Geometry: final body of the model. Coordinates: model frame, mm. Face numbers are marked on the shaded views. Give positions to 0.01 mm unless a question says otherwise; leave off trailing zeros. Write each loop counter-clockwise with the first axis right and the second up, starting at its lowest first coordinate (ties: lowest second). Pieces come first, ordered by that corner, then holes.
from build123d import *

# Parameters (mm, degrees)
F0_W     = 25.9
F0_H     = 9.85
F0_W_2   = 4.5
F0_H_2   = 4.5
F1_DEPTH = 5
F2_DEPTH = 4.08
F2_TAPER = 0.5
F3_W     = 3.15
F3_H     = 9.85
F4_DEPTH = 1
F5_R     = 2


with BuildPart() as f1:
    # F0 (on Front) → F1 (new body)
    with BuildSketch(Plane.XZ):
        with Locations((-28.4469606161, 4.925)):
            Rectangle(F0_W, F0_H)
        with Locations((-32.7639606161, 4.925)):
            Rectangle(F0_W_2, F0_H_2, mode=Mode.SUBTRACT)
        with Locations((-24.1299606161, 4.925)):
            Rectangle(F0_W_2, F0_H_2, mode=Mode.SUBTRACT)
        with Locations((-24.1299606161, 4.925)):
            Rectangle(F0_W_2, F0_H_2)
        with Locations((-32.7639606161, 4.925)):
            Rectangle(F0_W_2, F0_H_2)
    extrude(amount=F1_DEPTH)


with BuildPart() as f1b:
    # F0 (on Front) → F1, piece 2 (new body)
    with BuildSketch(Plane.XZ):
        with Locations((0.6030393839, 4.925)):
            Rectangle(F0_W, F0_H)
        with Locations((-3.7139606161, 4.925)):
            Rectangle(F0_W_2, F0_H_2, mode=Mode.SUBTRACT)
        with Locations((4.9200393839, 4.925)):
            Rectangle(F0_W_2, F0_H_2, mode=Mode.SUBTRACT)
        with Locations((4.9200393839, 4.925)):
            Rectangle(F0_W_2, F0_H_2)
        with Locations((-3.7139606161, 4.925)):
            Rectangle(F0_W_2, F0_H_2)
    extrude(amount=F1_DEPTH)


with BuildPart() as f2_tool:
    # F0 (on Front) → F2 (new body)
    with BuildSketch(Plane.XZ):
        with Locations((4.9200393839, 4.925)):
            Rectangle(F0_W_2, F0_H_2)
        with Locations((-3.7139606161, 4.925)):
            Rectangle(F0_W_2, F0_H_2)
        with Locations((-24.1299606161, 4.925)):
            Rectangle(F0_W_2, F0_H_2)
        with Locations((-32.7639606161, 4.925)):
            Rectangle(F0_W_2, F0_H_2)
    extrude(amount=F2_DEPTH, taper=F2_TAPER)


with BuildPart() as f1_1:
    add(f1.part)

    # F2: cut by f2_tool
    add(f2_tool.part, mode=Mode.SUBTRACT)



with BuildPart() as f1b_1:
    add(f1b.part)

    # F2: cut by f2_tool
    add(f2_tool.part, mode=Mode.SUBTRACT)


with BuildPart() as f1_2:
    add(f1_1.part)

    add(f1b_1.part)  # F4 merges F1b
    # F3 (on face) → F4 (join)
    with BuildSketch(Plane.XZ.offset(5)):
        with Locations((-13.9219606161, 4.925)):
            Rectangle(F3_W, F3_H)
    extrude(amount=-F4_DEPTH)

    # F5
    f5_edges = [f1_2.edges().sort_by_distance(p)[0] for p in [
        (-12.346961, 0, 4.925),
        (-15.496961, 0, 4.925),
        (13.553039, 0, 4.925),
        (-41.396961, 0, 4.925),
    ]]
    fillet(f5_edges, radius=F5_R)


solid = f1_2.part
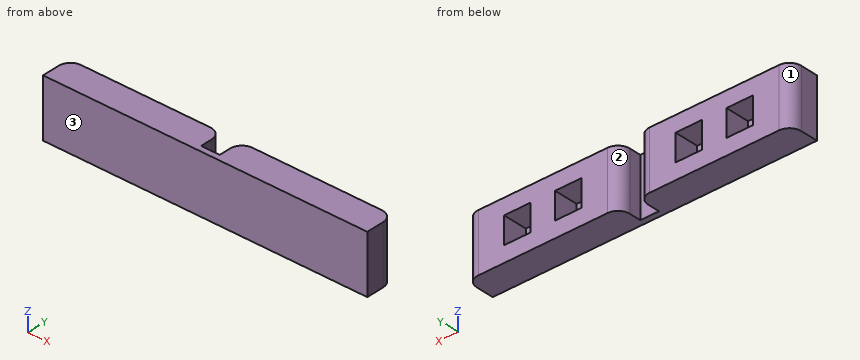
Q1. Pull-direction query (X, two-part tool) for the marked faces 1, 2 and 3; classes: released by +X, released by -X, zero draft, split by the parting line, or undercut.
Filled sheet:
face 1: released by -X
face 2: undercut
face 3: zero draft
Q2. Section C-C on x = -16.5. Output: boundary loops of the cut face in (y, z), plus the area to 3 significant figures.
Filled sheet:
outline: (-5, 0) - (-0.27, 0) - (-0.27, 9.85) - (-5, 9.85) - close
area: 46.6 mm2
Q3. Section A-A on z = 8. Output: boundary loops of the cut face in (x, y), plus the area to 3 significant figures.
Filled sheet:
outline: (-41.4, -5) - (13.55, -5) - (13.55, -2) arc R2 ccw to (11.55, 0) - (-10.35, 0) arc R2 ccw to (-12.35, -2) - (-12.35, -4) - (-15.5, -4) - (-15.5, -2) arc R2 ccw to (-17.5, 0) - (-39.4, 0) arc R2 ccw to (-41.4, -2) - close
area: 259 mm2
Q4. Pin query (flat end, axial travel): P1, Ø3.5, axis at x = -24, z = 5, coming from the +Y side; P2, Ø3.5, axis at x = -14.5, z = 6.5, coming from the +Y side. Return the tip coordinate at first contact, or that it passes through.
Filled sheet:
P1: stops at y = -4.08
P2: stops at y = -0.44
Q5. Section B-B on y = -0.85. Count the separate pieces of the cut face and the enclosed holes in it, plus the area to 3 significant figures.
Filled sheet:
separate pieces: 2
enclosed holes: 4
area: 415 mm2
Q6. Ray query, line 1 along X through (y, z) = (-2.75, 5); line 2 along X through (y, z) = (-3.9, 3); line 3 along X through (y, z) = (-2.1, 1.75). Return the intervals inside material, ascending.
Filled sheet:
line 1: x = -41.4 to -34.99, -30.54 to -26.36, -21.9 to -15.5, -12.35 to -5.94, -1.49 to 2.69, 7.15 to 13.55
line 2: x = -41.4 to -34.98, -30.55 to -26.35, -21.91 to -15.5, -12.35 to -5.93, -1.5 to 2.7, 7.14 to 13.55
line 3: x = -41.4 to -15.5, -12.35 to 13.55
